from build123d import *

# Parameters (mm, degrees)
SALIENTE_EXTRUIR1_DEPTH = 4
CROQUIS2_R              = 1.7
CORTAR_EXTRUIR1_DEPTH   = 4
CROQUIS3_R              = 2.95
CORTAR_EXTRUIR2_DEPTH   = 3


with BuildPart() as part:
    # Croquis1 → Saliente-Extruir1 (new body)
    with BuildSketch(Plane(origin=(0, 0, 0), x_dir=(1, 0, 0), z_dir=(0, 1, 0))):
        with BuildLine():
            Line((-7.200520814, 3.25), (-15, 3.25))
            Line((-15, 3.25), (-15, -3.25))
            Line((-15, -3.25), (-7.200520814, -3.25))
            ThreePointArc((-7.200520814, -3.25), (0, -7.9), (7.200520814, -3.25))
            Line((7.200520814, -3.25), (15, -3.25))
            Line((15, -3.25), (15, 3.25))
            Line((15, 3.25), (7.200520814, 3.25))
            ThreePointArc((7.200520814, 3.25), (0, 7.9), (-7.200520814, 3.25))
        make_face()
    extrude(amount=SALIENTE_EXTRUIR1_DEPTH)

    # Croquis2 → Cortar-Extruir1 (cut)
    with BuildSketch(Plane(origin=(0, 4, 0), x_dir=(1, 0, 0), z_dir=(0, 1, 0))):
        with Locations((-11, 0)):
            Circle(CROQUIS2_R)
        with Locations((11, 0)):
            Circle(CROQUIS2_R)
    extrude(amount=-CORTAR_EXTRUIR1_DEPTH, mode=Mode.SUBTRACT)

    # Croquis3 → Cortar-Extruir2 (cut)
    with BuildSketch(Plane(origin=(0, 4, 0), x_dir=(1, 0, 0), z_dir=(0, 1, 0))):
        with Locations((-11, 0)):
            Circle(CROQUIS3_R)
        with Locations((11, 0)):
            Circle(CROQUIS3_R)
    extrude(amount=-CORTAR_EXTRUIR2_DEPTH, mode=Mode.SUBTRACT)

    # Croquis4 → Cortar-Revolución1 (revolve, cut)
    with BuildSketch(Plane(origin=(0, 0, 0), x_dir=(0, 0, -1), z_dir=(1, 0, 0))):
        with BuildLine():
            Line((0, 4), (-10, 4))
            Line((-10, 4), (-10, 7))
            Line((-10, 7), (10, 7))
            Line((10, 7), (10, 3.083269132))
            ThreePointArc((10, 3.083269132), (5.02096593, 3.770337785), (0, 4))
        make_face()
    revolve(axis=Axis((0, -51, 21.725989645), (0, 0, -1)), mode=Mode.SUBTRACT)


solid = part.part
Can you work these out from the model? Positions are in its coordinate system, mm. A direction names the side the tool comes from. Give positions to 0.01 mm unless a question says otherwise; leave off trailing zeros. Loops run counter-clockwise (first coordinate to the right, second up) from the corner with the lowest first, then second, coordinate; pieces in that order, holes last. Notation, with made-up numbers: (5.5, 54) - (43.5, 54) arc R22 cw to (43.5, 61) - close; hole circle Ø1 at (80, 83). An arc over 180 degrees is marked (long way). Return JSON: item names as keys, results as strings.
1. I'm going to push flat-ended pins straight in: pin 1 Ø1.1 at (x, y) = (-10, 1) entering from +Z; pin 2 Ø3 at (x, z) = (-9.5, -0.5) entering from +Y; pin 3 Ø4.5 at (x, z) = (-11, 0) entering from +Y. Where does each tip first touch, or does it pass through?
Output values:
{"pin 1": "stops at z = 3.25", "pin 2": "stops at y = 3.41", "pin 3": "stops at y = 1"}
2. I want a section at B-B on z = -1. Give the number of separate pieces and of enclosed holes in the cut face, and give its area (3 significant figures).
Output values:
{"separate pieces": "3", "enclosed holes": "0", "area": "72.9 mm²"}
3. For faces 1 (the face through (11, 1, 3.25)), 2 (the face through (11, 1, 2)), 3 (the face through (-11, 1, -3.25)), which set-ups out of +Z, -Z, +X, -X, +Y, -Y let a thin tool reach every point of the face, with its end or its side?
Output values:
{"face 1": "+Z, +X, +Y, -Y", "face 2": "+Y", "face 3": "-Z, -X, +Y, -Y"}
4. I want a section at A-A on y = 1.45. Please give me the cut outline in (x, z).
Output values:
{"outline": "(-15, -3.25) - (-7.2, -3.25) arc R7.9 ccw to (7.2, -3.25) - (15, -3.25) - (15, 3.25) - (7.2, 3.25) arc R7.9 ccw to (-7.2, 3.25) - (-15, 3.25) - close; hole circle Ø5.9 at (-11, 0); hole circle Ø5.9 at (11, 0)"}
5. If I drill on line 1 (X direction, y = 0.45, z = 0); line 2 (Z direction, x = -11, y = 2.2); line 3 (X direction, y = 0.4, z = 0.75), over which ranges is the centre line in solid material (lowest first)?
Output values:
{"line 1": "x = -15 to -12.7, -9.3 to 9.3, 12.7 to 15", "line 2": "z = -3.25 to -2.95, 2.95 to 3.25", "line 3": "x = -15 to -12.53, -9.47 to 9.47, 12.53 to 15"}
